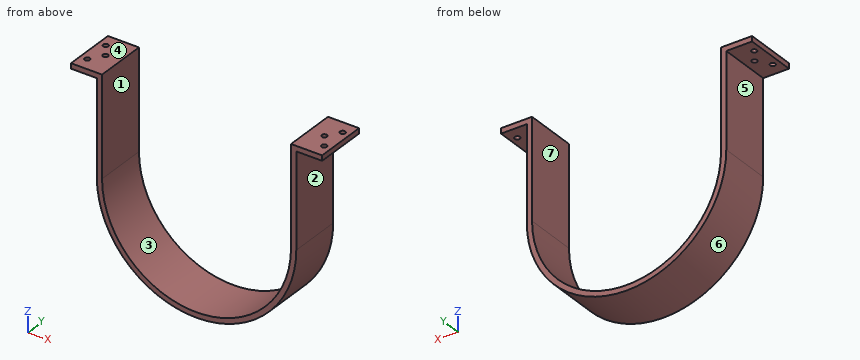
from build123d import *

# Parameters (mm, degrees)
BOSS_EXTRUDE1_DEPTH = 31.75
SKETCH15_R          = 3.175
CUT_EXTRUDE1_DEPTH  = 288.83021471


with BuildPart() as part:
    # Sketch1 → Boss-Extrude1 (new, symmetric)
    with BuildSketch(Plane(origin=(0, 0, 0), x_dir=(1, 0, 0), z_dir=(0, 1, 0))):
        with BuildLine():
            Line((-114.7, -121.05), (-114.7, 0))
            ThreePointArc((-114.7, 0), (0, 114.7), (114.7, 0))
            Line((114.7, 0), (114.7, -121.05))
            Line((114.7, -121.05), (152.4, -121.05))
            Line((152.4, -121.05), (152.4, -114.7))
            Line((152.4, -114.7), (121.05, -114.7))
            Line((121.05, -114.7), (121.05, 0))
            ThreePointArc((121.05, 0), (0, 121.05), (-121.05, 0))
            Line((-121.05, 0), (-121.05, -12.7))
            Line((-121.05, -12.7), (-121.05, -114.7))
            Line((-121.05, -114.7), (-152.4, -114.7))
            Line((-152.4, -114.7), (-152.4, -121.05))
            Line((-152.4, -121.05), (-114.7, -121.05))
        make_face()
    extrude(amount=BOSS_EXTRUDE1_DEPTH, both=True)

    # Sketch15 → Cut-Extrude1 (cut, through all)
    with BuildSketch(Plane.XY.offset(121.05)):
        with Locations((-143.76875, 15.875)):
            Circle(SKETCH15_R)
        with Locations((-143.76875, -15.875)):
            Circle(SKETCH15_R)
        with Locations((-132.85625, 0)):
            Circle(SKETCH15_R)
        with Locations(Location((132.85625, 0, 0), (0, 0, 180))):
            Circle(SKETCH15_R)
        with Locations((143.76875, -15.875)):
            Circle(SKETCH15_R)
        with Locations(Location((143.76875, 15.875, 0), (0, 0, 180))):
            Circle(SKETCH15_R)
    extrude(amount=-CUT_EXTRUDE1_DEPTH, mode=Mode.SUBTRACT)


solid = part.part
Geometry check sheet. Reference: the model listing, model coordinates, mm. Face numbers are marked on the shaded views. A direction names the side the tool comes from. Round coordinates to 2 decimals unless told otherwise and drop trailing zeros. Write each loop counter-clockwise with the first axis right and the second up, starting at its lowest first coordinate (ties: lowest second). Pieces come first, ordered by that corner, then holes.
Item 1: Access from +Z, -Z, +X, -X, +Y, -Y to the whole of each face (thin tool, end or side, straight path). Record for the marked faces 5, 6 and 7.
Determined:
face 5: -Z, -X, +Y, -Y
face 6: -Z, +Y, -Y
face 7: +Z, +Y, -Y
Item 2: Mould release check, pull along X, two halves, no side actions. Record for the marked faces 1, 2, 3 and 4: +X half, -X half, draft (parallel to the pull), parting line (faces both ways), or undercut.
Determined:
face 1: undercut
face 2: +X half
face 3: undercut
face 4: draft
Item 3: Section check B-B (z = 60.5). Record the boundary of the cut face in (x, y), plus the area to 3 significant figures.
Determined:
outline: (-121.05, -31.75) - (-114.7, -31.75) - (-114.7, 31.75) - (-121.05, 31.75) - close; (114.7, -31.75) - (121.05, -31.75) - (121.05, 31.75) - (114.7, 31.75) - close
area: 806 mm2
Item 4: Material ranges on line 1 along X through (y, z) = (29, 82.5); line 2 along X through (y, z) = (-9, -5); line 3 along Z through (x, y) = (-66.5, 16.5), recorded low to high.
Determined:
line 1: x = -121.05 to -114.7, 114.7 to 121.05
line 2: x = -120.95 to -114.59, 114.59 to 120.95
line 3: z = -101.15 to -93.46
Item 5: Go/stop test with flat-tipped pins: pin 1 Ø5 at (y, z) = (-7.5, 21.5) entering from +X; pin 2 Ø7.5 at (x, y) = (143.77, 15.88) entering from -Z; pin 3 Ø5.5 at (x, y) = (-143.77, 15.88) entering from +Z; pin 4 Ø7.5 at (x, y) = (143.77, -15.88) entering from +Z. Record where each tip stops, or that it passes through.
Determined:
pin 1: stops at x = 121.05
pin 2: stops at z = 114.7
pin 3: passes through
pin 4: stops at z = 121.05
Item 6: Section check A-A (y = 0). Record the boundary of the cut face in (x, z), plus the area to 3 significant figures.
Determined:
outline: (-152.4, 114.7) - (-136.03, 114.7) - (-136.03, 121.05) - (-152.4, 121.05) - close; (-129.68, 114.7) - (-121.05, 114.7) - (-121.05, 0) arc R121.05 ccw to (121.05, 0) - (121.05, 114.7) - (129.68, 114.7) - (129.68, 121.05) - (114.7, 121.05) - (114.7, 0) arc R114.7 cw to (-114.7, 0) - (-114.7, 121.05) - (-129.68, 121.05) - close; (136.03, 114.7) - (152.4, 114.7) - (152.4, 121.05) - (136.03, 121.05) - close
area: 4,210 mm2
Item 7: Section check D-D (x = 0). Record the boundary of the cut face in (y, z).
Determined:
outline: (-31.75, -121.05) - (31.75, -121.05) - (31.75, -114.7) - (-31.75, -114.7) - close
Item 8: Section check C-C (z = -23.5). Record the boundary of the cut face in (x, y), plus the area to 3 significant figures.
Determined:
outline: (-118.75, -31.75) - (-112.27, -31.75) - (-112.27, 31.75) - (-118.75, 31.75) - close; (112.27, -31.75) - (118.75, -31.75) - (118.75, 31.75) - (112.27, 31.75) - close
area: 823 mm2
